from build123d import *

# Parameters (mm, degrees)
SKETCH_1_R      = 13.5
EXTRUDE_1_DEPTH = 32


with BuildPart() as part:
    # 草图1 → 凸台-拉伸1 (new body)
    with BuildSketch(Plane(origin=(0, 0, 0), x_dir=(1, 0, 0), z_dir=(0, 0, -1))):
        Polygon((-120, 161), (-120, -137), (159, -137), (389.128205194, 438), (308.974573373, 497.794609338), align=None)
        with Locations(Location((0, 0, 0), (0, 0, 180))):
            Circle(SKETCH_1_R, mode=Mode.SUBTRACT)
        with Locations(Location((182.373558482, 244.468577054, 0), (0, 0, 180))):
            Circle(SKETCH_1_R, mode=Mode.SUBTRACT)
        with Locations(Location((230.209245953, 308.59148251, 0), (0, 0, 180))):
            Circle(SKETCH_1_R, mode=Mode.SUBTRACT)
        with Locations(Location((278.044933423, 372.714387967, 0), (0, 0, 180))):
            Circle(SKETCH_1_R, mode=Mode.SUBTRACT)
        with Locations(Location((325.880620894, 436.837293424, 0), (0, 0, 180))):
            Circle(SKETCH_1_R, mode=Mode.SUBTRACT)
        with Locations(Location((-80, 0, 0), (0, 0, 180))):
            Circle(SKETCH_1_R, mode=Mode.SUBTRACT)
        with Locations(Location((80, 0, 0), (0, 0, 180))):
            Circle(SKETCH_1_R, mode=Mode.SUBTRACT)
        with Locations(Location((-80, -80, 0), (0, 0, 180))):
            Circle(SKETCH_1_R, mode=Mode.SUBTRACT)
        with Locations(Location((0, -80, 0), (0, 0, 180))):
            Circle(SKETCH_1_R, mode=Mode.SUBTRACT)
        with Locations(Location((80, -80, 0), (0, 0, 180))):
            Circle(SKETCH_1_R, mode=Mode.SUBTRACT)
        with Locations(Location((-80, 80, 0), (0, 0, 180))):
            Circle(SKETCH_1_R, mode=Mode.SUBTRACT)
        with Locations(Location((0, 80, 0), (0, 0, 180))):
            Circle(SKETCH_1_R, mode=Mode.SUBTRACT)
        with Locations(Location((80, 80, 0), (0, 0, 180))):
            Circle(SKETCH_1_R, mode=Mode.SUBTRACT)
    extrude(amount=EXTRUDE_1_DEPTH)


solid = part.part
For this review, take the finished solid that the model builds, in its own axes (mm). Round coordinates to 2 decimals unless told otherwise and drop trailing zeros. Loops run counter-clockwise (first coordinate to the right, second up) from the corner with the lowest first, then second, coordinate; pieces in that order, holes last. Notation, with made-up numbers: (-30, 67.25) - (12, 67.25) arc R11 ccw to (12, 76.25) - close; hole circle Ø4 at (74.25, 88.5). An arc over 180 degrees is marked (long way). Answer as CSV lines item,"result".
(1) Mouldability with a two-part tool opening along Y and no side actions: class faces 1 (the face through (-66.513, 0.594, -15.776)), 2 (the face through (97.49, -331.755, -15.776)), 3 (the face through (18, 137, -16)) as +Y half, -Y half, draft (parallel to the pull), parting line (faces both ways), or undercut.
Checked values:
face 1,"undercut"
face 2,"-Y half"
face 3,"+Y half"
(2) Consider section D-D on x = 188. Give the boundary of the cut face in (y, z), then the cut area to 3 significant figures.
Checked values:
outline,"(-402.82, -32) - (-256.74, -32) - (-256.74, 0) - (-402.82, 0) - close; (-232.2, -32) - (64.54, -32) - (64.54, 0) - (-232.2, 0) - close"
area,"14,200 mm2"
(3) Consider section C-C on y = 80. Give the boundary of the cut face in (x, z).
Checked values:
outline,"(-120, -32) - (-93.5, -32) - (-93.5, 0) - (-120, 0) - close; (-66.5, -32) - (-13.5, -32) - (-13.5, 0) - (-66.5, 0) - close; (13.5, -32) - (66.5, -32) - (66.5, 0) - (13.5, 0) - close; (93.5, -32) - (181.81, -32) - (181.81, 0) - (93.5, 0) - close"
(4) Consider section A-A on x = -80. Give the boundary of the cut face in (y, z).
Checked values:
outline,"(-192.4, -32) - (-93.5, -32) - (-93.5, 0) - (-192.4, 0) - close; (-66.5, -32) - (-13.5, -32) - (-13.5, 0) - (-66.5, 0) - close; (13.5, -32) - (66.5, -32) - (66.5, 0) - (13.5, 0) - close; (93.5, -32) - (137, -32) - (137, 0) - (93.5, 0) - close"
(5) Consider section B-B on z = -22. Give the number of separate pieces and of enclosed holes in the cut face, then the cut area to 3 significant figures.
Checked values:
separate pieces,"1"
enclosed holes,"13"
area,"175,000 mm2"
(6) Insertion check: P1, Ø2, axis at y = -198.5, z = -8.5, coming from the +X side (3 decimals); P2, Ø10, axis at x = 87.5, y = -278, coming from the +Z side; P3, Ø12, axis at x = 240.5, z = -16, coming from the -Y side; P4, Ø16, axis at x = 0, y = 0, coming from the -Z side. Each pin has a flat end and moves straight along its axis. Give the tip position at first contact, or say it passes through.
Checked values:
P1,"stops at x = 293.675"
P2,"stops at z = 0"
P3,"stops at y = -448.74"
P4,"passes through"
(7) Wall thickness on line 1 (Y direction, x = -70, z = -28.5); line 2 (X direction, y = 72.5, z = -27); line 3 (Y direction, x = 0, z = -9): over which ranges is each line inside the solid? List them lowest first.
Checked values:
line 1,"y = -200.26 to -89.07, -70.93 to -9.07, 9.07 to 70.93, 89.07 to 137"
line 2,"x = -120 to -91.22, -68.78 to -11.22, 11.22 to 68.78, 91.22 to 184.81"
line 3,"y = -255.21 to -93.5, -66.5 to -13.5, 13.5 to 66.5, 93.5 to 137"
